Design review of the part built by this model. Coordinates are the model's own, in mm. A direction names the side the tool comes from. Give positions to 0.01 mm unless a question says otherwise; leave off trailing zeros. Write each loop counter-clockwise with the first axis right and the second up, starting at its lowest first coordinate (ties: lowest second). Pieces come first, ordered by that corner, then holes. Notation, with made-up numbers: (2, -37.75) -> (59, -37.75) arc R18 cw to (59, -27.75) -> close; hole circle Ø10 at (32.25, 64.5). An arc over 180 degrees is marked (long way). Answer as a JSON object with one key per item and string values.
Solid Edge part; units mm, degrees
sketch "Sketch1" plane through (0, 0, 0) normal (0, -1, 0) x (1, 0, 0)
  arc A0 (-7.4833, -13) -> (-7.4833, 13) centre (0, 0) cw
  line L0 (-7.4833, 13) -> (7.4833, 13)
  arc A1 (7.4833, 13) -> (7.4833, -13) centre (0, 0) cw
  line L1 (7.4833, -13) -> (-7.4833, -13)
  circle A2 centre (0, 0) radius 8
extrude "Protrusion1" add sketch "Sketch1" against normal blind 4.5
sketch "Sketch2" plane through (0, 0, 0) normal (0, -1, 0) x (1, 0, 0)
  line L0 (-7.4833, 13) -> (7.4833, 13)
  line L1 (-7.4833, -13) -> (7.4833, -13)
  arc A0 (-7.4833, -13) -> (-7.4833, 13) centre (0, 0) cw
  arc A1 (7.4833, 13) -> (7.4833, -13) centre (0, 0) cw
  circle A2 centre (0, 0) radius 7
extrude "ExtrudedProtrusion_2" add sketch "Sketch2" along normal blind 14
sketch "Sketch3" plane through (0, -14, 0) normal (0, -1, 0) x (1, 0, 0)
  line L0 (-7.4833, 13) -> (-22.0758, 4.6)
  line L1 (-22.0758, 4.6) -> (-22.0758, 1.6)
  line L2 (-22.0758, 1.6) -> (-30.9144, 1.6)
  line L3 (-30.9144, 1.6) -> (-30.9144, -1.6)
  line L4 (-22.0758, -1.6) -> (-30.9144, -1.6)
  line L5 (-22.0758, -4.6) -> (-22.0758, -1.6)
  line L6 (-7.4833, -13) -> (-22.0758, -4.6)
  line L7 (-7.4833, 13) -> (7.4833, 13)
extrude "Protrusion2" add sketch "Sketch3" against normal up to vertex (18.5 mm away) material side at (-14.7546, -14, 8.7567)
sketch "Sketch4" plane through (-2.3218, 4.5, 0) normal (0, 1, 0) x (-1, 0, 0)
  circle A0 centre (-13.3218, 0) radius 1.55
  circle A1 centre (8.6782, 0) radius 1.55
extrude "ExtrudedCutout_7" cut sketch "Sketch4" against normal blind 24
chamfer "Chamfer_4" distance 2 angle 45 1 edges at (-7, 0, 0) measured on face at (-5.1733, 0, -5.4933)
sketch "Sketch5" plane through (0, -4.75, -13) normal (0, 0, -1) x (0, -1, 0)
  circle A0 centre (5.25, 0) radius 1.625
extrude "ExtrudedCutout_10" cut sketch "Sketch5" against normal blind 36
sketch "Sketch6" plane through (-7.9572, -14, 0) normal (0, -1, 0) x (1, 0, 0)
  line L0 (-14.1186, 4.6) -> (0.4739, 13)
  line L1 (0.4739, 13) -> (15.4405, 13)
  line L2 (0.4265, -12.9726) -> (15.4405, -13)
  line L3 (-14.1186, -4.6) -> (0.4265, -12.9726)
  line L4 (-14.1186, -4.6) -> (-14.1186, -1.6)
  line L5 (-22.9572, -1.6) -> (-14.1186, -1.6)
  line L6 (-22.9572, -1.6) -> (-22.9572, 1.6)
  line L7 (-22.9572, 1.6) -> (-14.1186, 1.6)
  line L8 (-14.1186, 4.6) -> (-14.1186, 1.6)
  arc A0 (15.4405, 13) -> (15.4405, -13) centre (7.9572, 0) cw
  circle A1 centre (7.9572, 0) radius 7
extrude "ExtrudedProtrusion_7" add sketch "Sketch6" along normal blind 8
sketch "Sketch7" plane through (0, -8.75, 13) normal (0, 0, 1) x (0, 1, 0)
  line L0 (-13.25, 15.4833) -> (-13.25, 7.4833)
  line L1 (-13.25, 7.4833) -> (-13.25, -15)
  line L2 (-13.25, -15) -> (-5.25, -15)
  line L3 (-5.25, -15) -> (-5.25, 7.4833)
  line L4 (-5.25, 7.4833) -> (-13.25, 15.4833)
  line L5 (13.25, 14.9144) -> (-2.75, 30.9144)
  line L6 (-2.75, 30.9144) -> (13.25, 30.9144)
  line L7 (13.25, 30.9144) -> (13.25, 14.9144)
extrude "ExtrudedCutout_15" cut sketch "Sketch7" against normal blind 35.2747
sketch "Sketch8" plane through (-26.4951, -12.3307, 1.6) normal (0, 0, 1) x (1, 0, 0)
  circle A0 centre (0, -3.6193) radius 1.625
extrude "ExtrudedCutout_18" cut sketch "Sketch8" against normal blind 7.2202
sketch "Sketch9" plane through (-22.0758, -12.3307, -3.1025) normal (-1, 0, 0) x (0, -1, 0)
  line L0 (9.6693, 4.7025) -> (1.6693, 4.7025)
  line L1 (1.6693, 4.7025) -> (1.6693, 16.1025)
  line L2 (1.6693, 16.1025) -> (9.6693, 16.1025)
  line L3 (9.6693, 16.1025) -> (9.6693, 4.7025)
  line L4 (9.6693, 1.5025) -> (1.6693, 1.5025)
  line L5 (1.6693, 1.5025) -> (1.6693, -9.8975)
  line L6 (1.6693, -9.8975) -> (9.6693, -9.8975)
  line L7 (9.6693, -9.8975) -> (9.6693, 1.5025)
extrude "ExtrudedCutout_19" cut sketch "Sketch9" against normal blind 19.6868
(1) The part is to be moulded in two halves that separate along Z. For faces 1 (the flat face through (-22.076, -8, 3)), 2 (the flat face through (-14.677, -4.88, -8.859)), 3 (the cylindrical face through (12.55, -4.62, 0.07)), say which applies: +Z half, -Z half, draft (parallel to the pull), parting line (faces both ways), or undercut.
Here are the results:
{"face 1": "draft", "face 2": "-Z half", "face 3": "undercut"}
(2) We need section D-D, the plane y = 1.5. State the section outline as (x, z) points, then the cut area to 3 significant figures.
Here are the results:
{"outline": "(-17.91, -7) -> (-7.48, -13) -> (7.48, -13) arc R15 ccw to (7.48, 13) -> (-7.48, 13) -> (-17.91, 7) -> close; hole circle Ø3.1 at (-11, 0); hole circle Ø16 at (0, 0); hole circle Ø3.1 at (11, 0)", "area": "520 mm²"}
(3) Clearance check with flat-ended pins moving along their axes: pin 1 (3.5 mm diameter, centred on x = -11.5, z = -0.5, fed in from +Y); pin 2 (8 mm diameter, centred on x = -13, y = 0.5, fed in from +Z); pin 3 (6 mm diameter, centred on x = -22.5, y = -16.5, fed in from -Z); pin 4 (4 mm diameter, centred on x = -12.5, y = -8.5, fed in from -Z). State where each tip first meets the part, or that it passes through.
Here are the results:
{"pin 1": "stops at y = 4.5", "pin 2": "stops at z = 12.13", "pin 3": "stops at z = -5.31", "pin 4": "stops at z = -11.26"}
(4) We need section C-C, the plane x = 11. State the section outline as (y, z) points, then the cut area to 3 significant figures.
Here are the results:
{"outline": "(-14, -10.2) -> (4.5, -10.2) -> (4.5, -1.55) -> (-14, -1.55) -> close; (-14, 1.55) -> (4.5, 1.55) -> (4.5, 10.2) -> (-14, 10.2) -> close", "area": "320 mm²"}
(5) We need section B-B, the plane y = -10. State the section outline as (x, z) points (3 decimals), then the cut area to 3 significant figures.
Here are the results:
{"outline": "(-29.414, -1.6) -> (-22.076, -1.6) -> (-22.076, -4.6) -> (-7.483, -13) -> (-1.625, -13) -> (-1.625, -6.809) arc R7 cw to (-1.625, 6.809) -> (-1.625, 13) -> (-7.483, 13) -> (-22.076, 4.6) -> (-22.076, 1.6) -> (-29.414, 1.6) -> close; (1.625, -13) -> (7.483, -13) arc R15 ccw to (7.483, 13) -> (1.625, 13) -> (1.625, 6.809) arc R7 cw to (1.625, -6.809) -> close; hole circle Ø3.1 at (-11, 0); hole circle Ø3.1 at (11, 0)", "area": "600 mm²"}
(6) For line 1 along X through (y, z) = (0, -1); line 2 along Y through (x, z) = (0, 10.75) (3 decimals); line 3 along X through (y, z) = (2.75, 2.75), list the stretches that pass through material, from the lowest coordinate up.
Here are the results:
{"line 1": "x = -19.41 to -12.18, -9.82 to -7.94, 7.94 to 9.82, 12.18 to 14.97", "line 2": "y = -14 to -11.625, -8.375 to 4.5", "line 3": "x = -16.66 to -7.51, 7.51 to 14.75"}
(7) We need section A-A, the plane z = 0. State the section outline as (x, y) points (3 decimals), then the cut area to 3 significant figures.
Here are the results:
{"outline": "(-30.914, -22) -> (-15.483, -22) -> (-7.483, -14) -> (-7, -14) -> (-7, -2) -> (-8, -1) -> (-8, 4.5) -> (-9.45, 4.5) -> (-9.45, -14) -> (-12.55, -14) -> (-12.55, 4.5) -> (-14.914, 4.5) -> (-30.914, -11.5) -> close; (7, -14) -> (9.45, -14) -> (9.45, 4.5) -> (8, 4.5) -> (8, -1) -> (7, -2) -> close; (12.55, -14) -> (15, -14) -> (15, 4.5) -> (12.55, 4.5) -> close; hole circle Ø3.25 at (-26.495, -15.95)", "area": "483 mm²"}
(8) For faces 4 (the flat face through (-14.677, -4.88, 8.859)), 5 (the cylindrical face through (-9.77, -4.62, -0.94)), 6 (the flat face through (-22.076, -8, -3)), list the 3-axis set-ups (+Z, -Z, +X, -X, +Y, -Y) from which the entire face can be reached by the end or side of a thin tool; tool diameter is ignored.
Here are the results:
{"face 4": "+Z, -X, +Y, -Y", "face 5": "+Y", "face 6": "-Z, -X, +Y, -Y"}
